Work out the finished part from the listing and answer in its coordinate system (mm). Round coordinates to 2 decimals unless told otherwise and drop trailing zeros. Order: outer loops, then holes, each group sorted by start corner. A loop starts at its lowest first (then second) coordinate and runs counter-clockwise, first axis right, second up. Notation, with made-up numbers: (40.5, 39) -> (72.5, 39) arc R32 ccw to (72.5, 74) -> close; hole circle Ø5 at (-1, 88). An arc over 180 degrees is marked (long way). Use a Markdown table: item, result. Add a question column.
Item 1: A cutting plane is placed at C-C, the plane x = 320. Determine the outline of the cut face in (y, z), plus the area to 3 significant figures.
Item 2: Flat-ended cylindrical pins translate along their axes: P1, Ø1.5, axis at x = 187, y = -65, coming from the +Z side; P2, Ø4, axis at y = -13.5, z = -7.5, coming from the +X side. Find the tip coordinate at first contact, or state that the pin passes through.
Item 3: A cutting plane is placed at D-D, the plane y = -51. Determine the outline of the cut face in (x, z) (3 decimals), plus the area to 3 significant figures.
Item 4: Find the intervals of material crossed by L1, parallel to Z at x = 339, y = -42; L2, parallel to Y at x = 315, z = -3.5; L3, parallel to X at y = -11.5, z = -2.75, in increasing order. Write a range as [from, to].
Item 5: A cutting plane is placed at B-B, the plane z = -3.5. Determine the outline of the cut face in (x, y), plus the area to 3 significant figures.
from build123d import *

# Parameters (mm, degrees)
BOSS_EXTRUDE1_DEPTH = 82.55
SKETCH1_OUTSIDE_W   = 467.064
SKETCH1_OUTSIDE_H   = 163.534
CUT_EXTRUDE1_DEPTH  = 395.921504257
FILLET2_R           = 6.35
FILLET3_R           = 6.35


with BuildPart() as part:
    # Sketch2 → Boss-Extrude1 (new body)
    with BuildSketch(Plane(origin=(0, 0, 0), x_dir=(1, 0, 0), z_dir=(0, 1, 0))):
        Polygon((193.04, 9.525), (193.04, 0), (386.08, 0), (386.08, 6.35), (269.24, 9.525), align=None)
        Polygon((0, 6.35), (0, 0), (193.04, 0), (193.04, 9.525), (116.84, 9.525), align=None)
    extrude(amount=-BOSS_EXTRUDE1_DEPTH)

    # Sketch1 outside → Cut-Extrude1 (cut, through all)
    with BuildSketch(Plane.XY):
        with Locations((193.04, -41.275)):
            Rectangle(SKETCH1_OUTSIDE_W, SKETCH1_OUTSIDE_H)
        Polygon((0, 0), (386.08, 0), (386.08, -46.228), (231.14, -82.55), (154.94, -82.55), (0, -46.228), align=None, mode=Mode.SUBTRACT)
    extrude(amount=-CUT_EXTRUDE1_DEPTH, mode=Mode.SUBTRACT)

    # Fillet2
    fillet2_edges = [part.edges().sort_by_distance(p)[0] for p in [
        (386.08, -23.114, -6.35),
    ]]
    fillet(fillet2_edges, radius=FILLET2_R)

    # Fillet3
    fillet3_edges = [part.edges().sort_by_distance(p)[0] for p in [
        (0, -23.114, -6.35),
    ]]
    fillet(fillet3_edges, radius=FILLET3_R)


solid = part.part
Reported:
| question | item | result |
|---|---|---|
| 1 | outline | (-61.72, -8.15) -> (0, -8.15) -> (0, 0) -> (-61.72, 0) -> close |
| 1 | area | 503 mm² |
| 2 | P1 | z = 0 |
| 2 | P2 | x = 383.18 |
| 3 | outline | (20.356, -6.903) -> (116.84, -9.525) -> (269.24, -9.525) -> (365.724, -6.903) -> (365.724, 0) -> (20.356, 0) -> close |
| 3 | area | 3,040 mm² |
| 4 | L1 | [-7.63, 0] |
| 4 | L2 | [-62.89, 0] |
| 4 | L3 | [0.55, 385.53] |
| 5 | outline | (0.94, -46.45) -> (154.94, -82.55) -> (231.14, -82.55) -> (385.14, -46.45) -> (385.14, 0) -> (0.94, 0) -> close |
| 5 | area | 26,200 mm² |
